Read the model definition and answer for the solid it produces. Units are mm, in the model's axes. A direction names the side the tool comes from. Coordinates: 2 decimals unless noted, no trailing zeros. Order: outer loops, then holes, each group sorted by start corner. A loop starts at its lowest first (then second) coordinate and runs counter-clockwise, first axis right, second up. Notation, with made-up numbers: M -25,80 L -9,80 A31 ccw -9,112 Z; hole C -2.5,-30 d3. An arc over 180 degrees is marked long. Use a Markdown table: item, result. Add a question column.
1) Find section D-D on x = -13. Write down the section's boundary in (y, z), plus the area to 3 significant figures.
2) Find the intervals of material crossed by probe 1 along Y at (x, z) = (0, 5.5); probe 2 along Z at (x, y) = (-0.5, -5.5); probe 3 along X at (y, z) = (12, 3), in increasing order. Write a range as [from, to].
3) Find section C-C on y = 13.5. Write down the section's boundary in (x, z).
4) Each of these flat-tipped pins is pushed along its axis until it touches: pin 1 Ø4 at (x, y) = (0, -11.52) entering from -Z; pin 2 Ø1.5 at (x, y) = (3, -7) entering from +Z; pin 3 Ø1 at (y, z) = (3, 3) entering from +X. Where does it stop, or does it pass through?
5) For faces 4 (the face through (-1.08, -4.88, 7.04)), 5 (the face through (6.801, -6.035, 2.028)), determine the directions among +Z, -Z, +X, -X, +Y, -Y from which every point of the face is accessible in a straight line to the end or side of a thin tool.
6) The mould has two halves that part along X. Classify faces 1 (the face through (-4, 4, 4)), 2 (the face through (-0.867, -3.905, 4.93)), 3 (the face through (-3.47, -15.62, 1.97)): released by +X, released by -X, zero draft, split by the parting line, or undercut.
7) Find section A-A on x = 0. Write down the section's boundary in (y, z), plus the area to 3 significant figures.
from build123d import *

# Parameters (mm, degrees)
SKETCH_1_R               = 16
SKETCH_1_R_2             = 4
EXTRUDE_2_DEPTH          = 10
SKETCH_3_R               = 16
SKETCH_3_R_2             = 5
CUT_EXTRUDE_2_DEPTH      = 6
SKETCH_4_R               = 2.5
CUT_EXTRUDE_3_DEPTH      = 5
PATTERN_CIRCULAR_1_COUNT = 8


with BuildPart() as part:
    # 草图1 → 凸台-拉伸2 (new body)
    with BuildSketch(Plane.XY):
        Circle(SKETCH_1_R)
        Circle(SKETCH_1_R_2, mode=Mode.SUBTRACT)
    extrude(amount=EXTRUDE_2_DEPTH)

    # 草图3 → 切除-拉伸2 (cut)
    with BuildSketch(Plane.XY.offset(10)):
        Circle(SKETCH_3_R)
        Circle(SKETCH_3_R_2, mode=Mode.SUBTRACT)
    extrude(amount=-CUT_EXTRUDE_2_DEPTH, mode=Mode.SUBTRACT)

    # 草图4 → 切除-拉伸3 (cut, through all)
    with BuildSketch(Plane.XY.offset(4)):
        with Locations((0, 11.516849164)):
            Circle(SKETCH_4_R)
    cut_extrude_3 = extrude(amount=-CUT_EXTRUDE_3_DEPTH, mode=Mode.SUBTRACT)

    # 阵列(圆周)1: 切除-拉伸3 ×8 about axis
    pattern_circular_1_axis = Axis((0, 0, 0), (0, 0, 1))
    for i in range(1, PATTERN_CIRCULAR_1_COUNT):
        add(cut_extrude_3.rotate(pattern_circular_1_axis, i * 360 / PATTERN_CIRCULAR_1_COUNT), mode=Mode.SUBTRACT)


solid = part.part
Check result:
| question | item | result |
|---|---|---|
| 1 | outline | M -9.33,0 L -2.01,0 L -2.01,4 L -9.33,4 Z; M 2.01,0 L 9.33,0 L 9.33,4 L 2.01,4 Z |
| 1 | area | 58.5 mm2 |
| 2 | probe 1 | y = [-5, -4], [4, 5] |
| 2 | probe 2 | z = [0, 4] |
| 2 | probe 3 | x = [-10.58, -2.45], [2.45, 10.58] |
| 3 | outline | M -8.59,0 L -1.52,0 L -1.52,4 L -8.59,4 Z; M 1.52,0 L 8.59,0 L 8.59,4 L 1.52,4 Z |
| 4 | pin 1 | passes through |
| 4 | pin 2 | stops at z = 4 |
| 4 | pin 3 | stops at x = 15.8 |
| 5 | face 4 | +Z |
| 5 | face 5 | +Z, -Z |
| 6 | face 1 | zero draft |
| 6 | face 2 | undercut |
| 6 | face 3 | split by the parting line |
| 7 | outline | M -16,0 L -14.02,0 L -14.02,4 L -16,4 Z; M -9.02,0 L -4,0 L -4,10 L -5,10 L -5,4 L -9.02,4 Z; M 4,0 L 9.02,0 L 9.02,4 L 5,4 L 5,10 L 4,10 Z; M 14.02,0 L 16,0 L 16,4 L 14.02,4 Z |
| 7 | area | 68.0 mm2 |
